from build123d import *

# Parameters (mm, degrees)
PAD009_DEPTH    = 20
SKETCH027_R     = 8.2
POCKET015_DEPTH = 30
SKETCH028_R     = 8.2
POCKET016_DEPTH = 30
SKETCH031_R     = 1.6
POCKET018_DEPTH = 5
FILLET006_R     = 5


with BuildPart() as part:
    # Sketch026 → Pad009 (new body)
    with BuildSketch(Plane.XY):
        Polygon((-20, 20), (-20, -30), (0, -30), (0, 0), (30, 0), (30, 20), align=None)
    extrude(amount=PAD009_DEPTH)

    # Sketch027 → Pocket015 (cut)
    with BuildSketch(Plane.XZ.offset(30)):
        with Locations((-10, 10)):
            Circle(SKETCH027_R)
    extrude(amount=-POCKET015_DEPTH, mode=Mode.SUBTRACT)

    # Sketch028 → Pocket016 (cut)
    with BuildSketch(Plane.YZ.offset(30)):
        with Locations((10, 10)):
            Circle(SKETCH028_R)
    extrude(amount=-POCKET016_DEPTH, mode=Mode.SUBTRACT)

    # Sketch031 → Pocket018 (cut)
    with BuildSketch(Plane.XY.offset(20)):
        with Locations((20, 10)):
            Circle(SKETCH031_R)
        with Locations((-10, -20)):
            Circle(SKETCH031_R)
    extrude(amount=-POCKET018_DEPTH, mode=Mode.SUBTRACT)

    # Fillet006
    fillet006_edges = [part.edges().sort_by_distance(p)[0] for p in [
        (15, 0, 20),
        (0, -15, 20),
        (-20, -5, 20),
        (5, 20, 20),
        (5, 20, 0),
        (-20, 20, 10),
        (-20, -5, 0),
        (0, -15, 0),
        (15, 0, 0),
        (0, 0, 10),
    ]]
    fillet(fillet006_edges, radius=FILLET006_R)


solid = part.part
Input: part model. Units: mm. Frame: model coordinates. A direction names the side the tool comes from. Coordinates: 2 decimals unless noted, no trailing zeros. Loops run counter-clockwise (first coordinate to the right, second up) from the corner with the lowest first, then second, coordinate; pieces in that order, holes last.
Q1. Cut plane B-B (x = 27.5). Output: boundary loops of the cut face in (y, z), then the cut area to 3 significant figures.
Q2. Draft query along X for faces 1 (the face through (-2, -17, 19)), 2 (the face through (-10, 0, 10)), 3 (the face through (18, 2, 19)). Return one class per face: +X half, -X half, draft (parallel to the pull), parting line (faces both ways), or undercut.
Q3. Cut plane C-C (y = -13). Output: boundary loops of the cut face in (x, z), then the cut area to 3 significant figures.
Q4. Cut plane A-A (x = -10). Output: boundary loops of the cut face in (y, z), then the cut area to 3 significant figures.
Q5. Set-up query: faces 4 (the face through (-6.216, -15.21, 2.725)), 5 (the face through (15.21, 13.784, 2.725)), 6 (the face through (18, 2, 1)), 7 (the face through (18.4, 10.07, 19.03)). Return all of +Z, -Z, +X, -X, +Y, -Y with unobstructed straight access to the full face (end or side cutting, diameter ignored); none if empty.
Q6. Material intervals for line 1 (Z direction, x = 24, y = 10); line 2 (Y direction, x = -12.5, z = 12.5); line 3 (Y direction, x = 2, z = 11.75), sorted ascending.
Q7. Cut plane D-D (z = 10). Output: boundary loops of the cut face in (x, y), then the cut area to 3 significant figures.
Q8. Contact query for flat-ended pins moving along their axis: pin 1 (5 mm diameter, centred on x = -12.5, z = 9.5, fed in from -Y); pin 2 (3 mm diameter, centred on x = -3, y = -20.5, fed in from -Z); pin 3 (3 mm diameter, centred on x = 20, y = 10, fed in from +Z). Output: stop coordinate, or through.
Working result:
1. outline: (0, 5) arc R5 ccw to (5, 0) - (15, 0) arc R5 ccw to (20, 5) - (20, 15) arc R5 ccw to (15, 20) - (5, 20) arc R5 ccw to (0, 15) - close; hole circle Ø16.4 at (10, 10)
1. area: 167 mm2
2. face 1: +X half
2. face 2: undercut
2. face 3: draft
3. outline: (-20, 5) arc R5 ccw to (-15, 0) - (-5, 0) arc R5 ccw to (0, 5) - (0, 15) arc R5 ccw to (-5, 20) - (-15, 20) arc R5 ccw to (-20, 15) - close; hole circle Ø16.4 at (-10, 10)
3. area: 167 mm2
4. outline: (-30, 0) - (15, 0) arc R5 ccw to (20, 5) - (20, 15) arc R5 ccw to (15, 20) - (-18.4, 20) - (-18.4, 18.2) - (0, 18.2) - (0, 1.8) - (-30, 1.8) - close; (-30, 18.2) - (-21.6, 18.2) - (-21.6, 20) - (-30, 20) - close
4. area: 492 mm2
5. face 4: -Y
5. face 5: +X
5. face 6: -Z, +X, -Y
5. face 7: +Z
6. line 1: z = 0 to 1.8, 18.2 to 20
6. line 2: y = 0 to 20
6. line 3: y = -1 to 1.99, 18.01 to 20
7. outline: (-20, -30) - (-18.2, -30) - (-18.2, 0) - (-1.8, 0) - (-1.8, -30) - (0, -30) - (0, -5) arc R5 cw to (5, 0) - (30, 0) - (30, 1.8) - (0, 1.8) - (0, 18.2) - (30, 18.2) - (30, 20) - (-15, 20) arc R5 ccw to (-20, 15) - close
7. area: 616 mm2
8. pin 1: stops at y = 0
8. pin 2: stops at z = 0.03
8. pin 3: stops at z = 1.94
